Here's the drawing with two shaded views (mm, measured from the low corner). I have some questions. Round coordinates to 2 decimals unless told otherwise and drop trailing zeros. Loops run counter-clockwise (first coordinate to the right, second up) from the corner with the lowest first, then second, coordinate; pieces in that order, holes last.
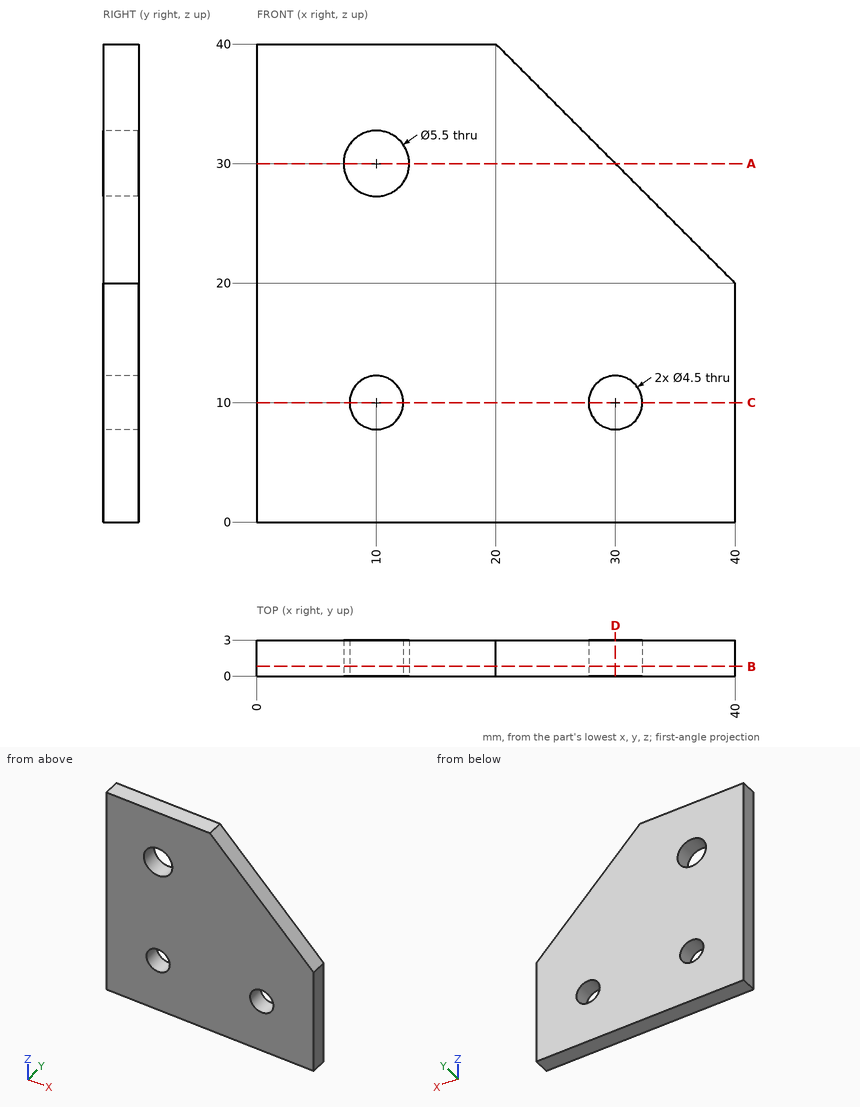
Item 1: Will this pin go through, and if not, where does the flat tip stop? pin 1 (2 mm diameter, centred on x = 10.5, z = 9.5, fed in from +Y).
Results list:
pin 1: passes through
Item 2: If we section it at D-D, the plane x = 30: Please give me the cut outline in (y, z).
Results list:
outline: (0, 0) - (3, 0) - (3, 7.75) - (0, 7.75) - close; (0, 12.25) - (3, 12.25) - (3, 30) - (0, 30) - close
Item 3: If we section it at C-C, the plane z = 10: Please give me the cut outline in (x, y), then the cut area to 3 significant figures.
Results list:
outline: (0, 0) - (7.75, 0) - (7.75, 3) - (0, 3) - close; (12.25, 0) - (27.75, 0) - (27.75, 3) - (12.25, 3) - close; (32.25, 0) - (40, 0) - (40, 3) - (32.25, 3) - close
area: 93.0 mm2
Item 4: If I drill on line 1 along X through (y, z) = (1.8, 10); line 2 along Z through (x, y) = (10, 1.7); line 3 along Z through (x, y) = (8, 0.65), over which ranges is the centre line in solid material (lowest first)?
Results list:
line 1: x = 0 to 7.75, 12.25 to 27.75, 32.25 to 40
line 2: z = 0 to 7.75, 12.25 to 27.25, 32.75 to 40
line 3: z = 0 to 8.97, 11.03 to 28.11, 31.89 to 40
Item 5: If we section it at A-A, the plane z = 30: Please give me the cut outline in (x, y), then the cut area to 3 significant figures.
Results list:
outline: (0, 0) - (7.25, 0) - (7.25, 3) - (0, 3) - close; (12.75, 0) - (30, 0) - (30, 3) - (12.75, 3) - close
area: 73.5 mm2
Item 6: If we section it at B-B, the plane y = 0.8: Please give me the cut outline in (x, z).
Results list:
outline: (0, 0) - (40, 0) - (40, 20) - (20, 40) - (0, 40) - close; hole circle Ø5.5 at (10, 30); hole circle Ø4.5 at (10, 10); hole circle Ø4.5 at (30, 10)
